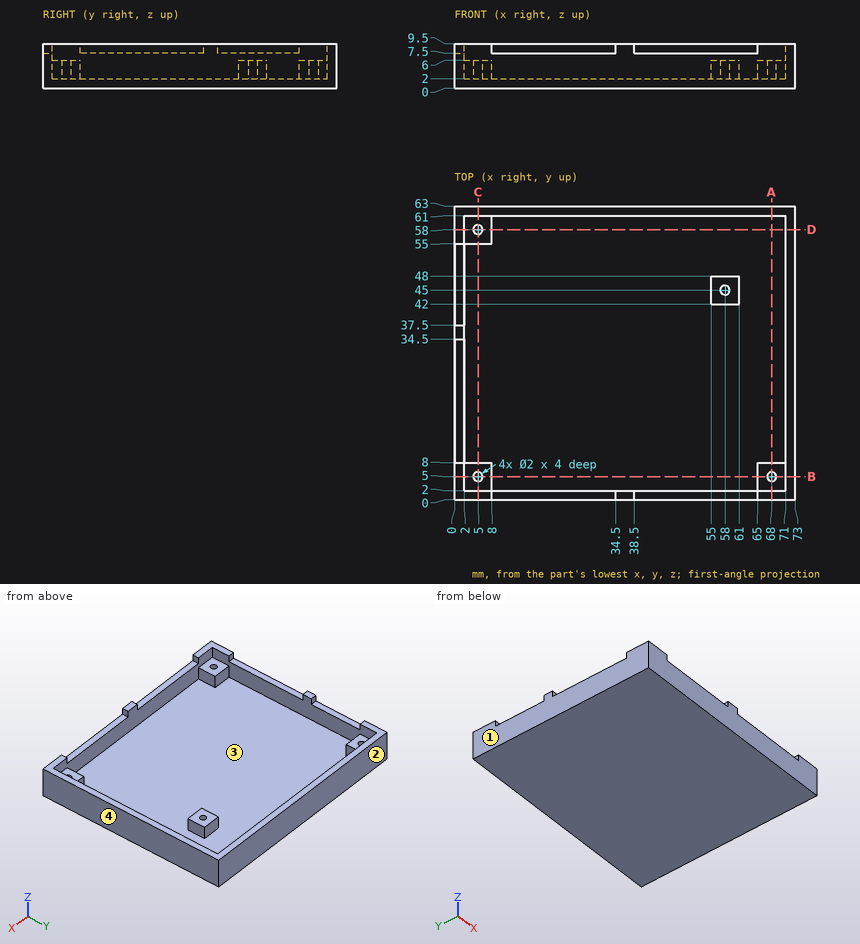
The figure shows three views and two pictorial views of one solid part (mm, origin at its lowest corner). Answer the questions. Coordinates: 2 decimals unless noted, no trailing zeros. Order: outer loops, then holes, each group sorted by start corner. A loop starts at its lowest first (then second) coordinate and runs counter-clockwise, first axis right, second up. Notation, with made-up numbers: (-17, 22.25) - (-4, 22.25) arc R18 ccw to (-4, 26.25) - close; hole circle Ø9 at (87.5, 21). An arc over 180 degrees is marked (long way). Answer as a JSON object with one key per item and string values.
1. Find section A-A on x = 68. Determine the outline of the cut face in (y, z).
Output values:
{"outline": "(0, 0) - (63, 0) - (63, 9.5) - (61, 9.5) - (61, 2) - (8, 2) - (8, 6) - (6, 6) - (6, 2) - (4, 2) - (4, 6) - (2, 6) - (2, 9.5) - (0, 9.5) - close"}
2. Consider line 1 (Y direction, x = 58, z = 4.5); line 2 (X direction, y = 45, z = 3.35); line 3 (X direction, y = 43, z = 2.75). Determine where each line is inside the solid, lowest interval first.
Output values:
{"line 1": "y = 0 to 2, 42 to 44, 46 to 48, 61 to 63", "line 2": "x = 0 to 2, 55 to 57, 59 to 61, 71 to 73", "line 3": "x = 0 to 2, 55 to 61, 71 to 73"}
3. The mould has two halves that part along X. Classify the marked faces 1, 2, 3 and 4: +X half, -X half, draft (parallel to the pull), parting line (faces both ways), or undercut.
Output values:
{"face 1": "-X half", "face 2": "draft", "face 3": "undercut", "face 4": "+X half"}
4. Find section D-D on y = 58. Determine the outline of the cut face in (x, z).
Output values:
{"outline": "(0, 0) - (73, 0) - (73, 9.5) - (71, 9.5) - (71, 2) - (8, 2) - (8, 6) - (6, 6) - (6, 2) - (4, 2) - (4, 6) - (2, 6) - (2, 9.5) - (0, 9.5) - close"}
5. Each of these flat-tipped pins is pushed along its axis until it touches: P1, Ø1.5, axis at x = 30.5, z = 6, coming from the -Y side; P2, Ø3, axis at x = 6, y = 58, coming from the +Z side; P3, Ø0.6, axis at x = 1, y = 23.5, coming from the +Z side; P4, Ø1.6, axis at x = 58, y = 45, coming from the +Z side. Where does it stop, or does it pass through?
Output values:
{"P1": "stops at y = 0", "P2": "stops at z = 6", "P3": "stops at z = 7.5", "P4": "stops at z = 2"}
6. Find section B-B on y = 5. Determine the outline of the cut face in (x, z).
Output values:
{"outline": "(0, 0) - (73, 0) - (73, 9.5) - (71, 9.5) - (71, 6) - (69, 6) - (69, 2) - (67, 2) - (67, 6) - (65, 6) - (65, 2) - (8, 2) - (8, 6) - (6, 6) - (6, 2) - (4, 2) - (4, 6) - (2, 6) - (2, 9.5) - (0, 9.5) - close"}
7. Find section C-C on x = 5. Determine the outline of the cut face in (y, z), plus the area to 3 significant figures.
Output values:
{"outline": "(0, 0) - (63, 0) - (63, 9.5) - (61, 9.5) - (61, 6) - (59, 6) - (59, 2) - (57, 2) - (57, 6) - (55, 6) - (55, 2) - (8, 2) - (8, 6) - (6, 6) - (6, 2) - (4, 2) - (4, 6) - (2, 6) - (2, 9.5) - (0, 9.5) - close", "area": "188 mm²"}
